```python
from build123d import *

# Parameters (mm, degrees)
BOSS_EXTRUDE1_DEPTH     = 50
SKETCH2_W               = 70
SKETCH2_H               = 26.5
CUT_EXTRUDE1_DEPTH      = 1
CUT_EXTRUDE1_DEPTH_BACK = 26
FILLET1_R               = 2.5
FILLET2_R               = 5
SKETCH3_R               = 1.6
CUT_EXTRUDE2_DEPTH      = 23.0000001
CUT_EXTRUDE2_DEPTH_BACK = 4


with BuildPart() as part:
    # Sketch1 → Boss-Extrude1 (new body, symmetric)
    with BuildSketch(Plane(origin=(0, 0, 0), x_dir=(0, 0, -1), z_dir=(1, 0, 0))):
        with BuildLine():
            Line((-11, 11.5), (11, 11.5))
            ThreePointArc((11, 11.5), (19.131727984, 8.131727984), (22.5, 0))
            Line((22.5, 0), (22.5, -11.5))
            Line((22.5, -11.5), (34.5, -11.5))
            Line((34.5, -11.5), (34.5, -8.5))
            Line((34.5, -8.5), (25, -8.5))
            Line((25, -8.5), (25, 0))
            Line((25, 0), (25, 3.5))
            ThreePointArc((25, 3.5), (22.071067812, 10.571067812), (15, 13.5))
            Line((15, 13.5), (-15, 13.5))
            ThreePointArc((-15, 13.5), (-22.071067812, 10.571067812), (-25, 3.5))
            Line((-25, 3.5), (-25, 0))
            Line((-25, 0), (-25, -8.5))
            Line((-25, -8.5), (-34.5, -8.5))
            Line((-34.5, -8.5), (-34.5, -11.5))
            Line((-34.5, -11.5), (-22.5, -11.5))
            Line((-22.5, -11.5), (-22.5, 0))
            ThreePointArc((-22.5, 0), (-19.131727984, 8.131727984), (-11, 11.5))
        make_face()
    extrude(amount=BOSS_EXTRUDE1_DEPTH, both=True)

    # Sketch2 → Cut-Extrude1 (cut, two sides)
    with BuildSketch(Plane(origin=(0, 13.5, 0), x_dir=(1, 0, 0), z_dir=(0, 1, 0))) as cut_extrude1_sk:
        with Locations((0, 21.25)):
            Rectangle(SKETCH2_W, SKETCH2_H)
        with Locations((0, -21.25)):
            Rectangle(SKETCH2_W, SKETCH2_H)
    extrude(amount=CUT_EXTRUDE1_DEPTH, mode=Mode.SUBTRACT)
    extrude(cut_extrude1_sk.sketch, amount=-CUT_EXTRUDE1_DEPTH_BACK, mode=Mode.SUBTRACT)

    # Fillet1
    fillet1_edges = [part.edges().sort_by_distance(p)[0] for p in [
        (42.5, -8.5, 25),
        (42.5, -8.5, -25),
        (-42.5, -8.5, 25),
        (-42.5, -8.5, -25),
    ]]
    fillet(fillet1_edges, radius=FILLET1_R)

    # Fillet2
    fillet2_edges = [part.edges().sort_by_distance(p)[0] for p in [
        (35, 12.5, -8),
        (35, 12.5, 8),
        (-35, 12.5, 8),
        (-35, 12.5, -8),
    ]]
    fillet(fillet2_edges, radius=FILLET2_R)

    # Sketch3 → Cut-Extrude2 (cut, two sides)
    with BuildSketch(Plane(origin=(0, -8.5, 0), x_dir=(1, 0, 0), z_dir=(0, 1, 0))) as cut_extrude2_sk:
        with Locations((42.5, -31)):
            Circle(SKETCH3_R)
        with Locations((42.5, 31)):
            Circle(SKETCH3_R)
        with Locations((-42.5, 31)):
            Circle(SKETCH3_R)
        with Locations((-42.5, -31)):
            Circle(SKETCH3_R)
    extrude(amount=CUT_EXTRUDE2_DEPTH, mode=Mode.SUBTRACT)
    extrude(cut_extrude2_sk.sketch, amount=-CUT_EXTRUDE2_DEPTH_BACK, mode=Mode.SUBTRACT)


solid = part.part
```
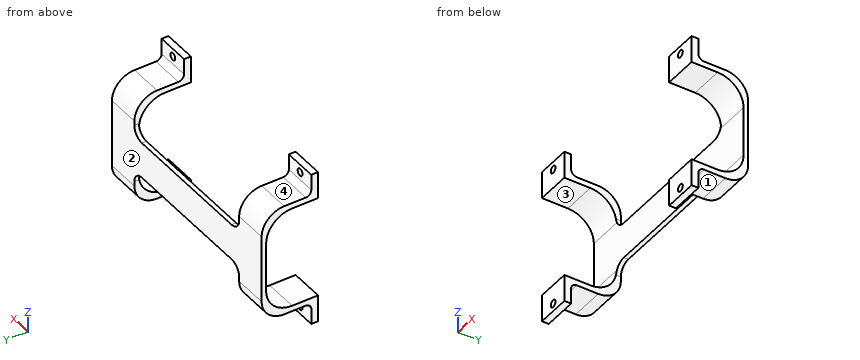
Can you work these out from the model? Positions are in its coordinate system, mm. Face numbers are marked on the shaded views. A direction names the side the tool comes from. Give positions to 0.01 mm unless a question says otherwise; leave off trailing zeros. Loops run counter-clockwise (first coordinate to the right, second up) from the corner with the lowest first, then second, coordinate; pieces in that order, holes last. Notation, with made-up numbers: M 38.25,-23 L 88.25,-23 A12 cw 88.25,-5 Z; hole C 48.5,89 d3. An arc over 180 degrees is marked long. Answer in a Markdown table with one row per item.
1. Suppose I cut it at D-D on x = 38. Write out the boundary of the cut face in (y, z).
Taken from the geometry:
| item | result |
|---|---|
| outline | M -11.5,-34.5 L -8.5,-34.5 L -8.5,-27.5 A2.5 cw -6,-25 L 3.5,-25 A10 ccw 13.5,-15 L 13.5,15 A10 ccw 3.5,25 L -6,25 A2.5 cw -8.5,27.5 L -8.5,34.5 L -11.5,34.5 L -11.5,22.5 L 0,22.5 A11.5 cw 11.5,11 L 11.5,-11 A11.5 cw 0,-22.5 L -11.5,-22.5 Z |
2. Suppose I cut it at C-C on y = -2.25. Write out the boundary of the cut face in (x, z), plus the area to 3 significant figures.
Taken from the geometry:
| item | result |
|---|---|
| outline | M -50,-25 L -35,-25 L -35,-22.5 L -50,-22.5 Z; M -50,22.5 L -35,22.5 L -35,25 L -50,25 Z; M 35,-25 L 50,-25 L 50,-22.5 L 35,-22.5 Z; M 35,22.5 L 50,22.5 L 50,25 L 35,25 Z |
| area | 150 mm² |
3. If I drill on line 1 along Z through (x, y) = (-42.5, -10); line 2 along X through (y, z) = (-10.3, 31); line 3 along X through (y, z) = (-2, 24), over which ranges is the centre line in solid material (lowest first)?
Taken from the geometry:
| item | result |
|---|---|
| line 1 | z = -34.5 to -32.6, -29.4 to -22.5, 22.5 to 29.4, 32.6 to 34.5 |
| line 2 | x = -50 to -44.1, -40.9 to -35, 35 to 40.9, 44.1 to 50 |
| line 3 | x = -50 to -35, 35 to 50 |
4. Suppose I cut it at B-B on z = -31. Write out the boundary of the cut face in (x, y), plus the area to 3 significant figures.
Taken from the geometry:
| item | result |
|---|---|
| outline | M -50,-11.5 L -44.1,-11.5 L -44.1,-8.5 L -50,-8.5 Z; M -40.9,-11.5 L -35,-11.5 L -35,-8.5 L -40.9,-8.5 Z; M 35,-11.5 L 40.9,-11.5 L 40.9,-8.5 L 35,-8.5 Z; M 44.1,-11.5 L 50,-11.5 L 50,-8.5 L 44.1,-8.5 Z |
| area | 70.8 mm² |
5. For pin 1 Ø3.5 at (x, z) = (-42, -32.5) entering from +Y; pin 2 Ø10 at (x, y) = (-39.5, -1.5) entering from +Z; pin 3 Ø5 at (x, y) = (-42.5, 0) entering from -Z; pin 4 Ø12 at (x, z) = (1, 15.5) entering from -Y, each with a flat end and sliding along its axis, tell me the tip position at first contact or that it passes through.
Taken from the geometry:
| item | result |
|---|---|
| pin 1 | stops at y = -8.5 |
| pin 2 | stops at z = 25.05 |
| pin 3 | stops at z = -25 |
| pin 4 | passes through |
6. Which directions (+Z, -Z, +X, -X, +Y, -Y) give clear straight access to the entire face, cutting with the end or side of a thin tool? Please do the marked faces 1, 2, 3 and 4.
Taken from the geometry:
| item | result |
|---|---|
| face 1 | -Z, +X, -X, +Y |
| face 2 | +Z, -Z, +X, -X, +Y |
| face 3 | +X, -X, -Y |
| face 4 | +Z, +X, -X, +Y |
7. Suppose I cut it at A-A on x = -42.5. Write out the boundary of the cut face in (y, z), plus the area to 3 significant figures.
Taken from the geometry:
| item | result |
|---|---|
| outline | M -11.5,-34.5 L -8.5,-34.5 L -8.5,-32.6 L -11.5,-32.6 Z; M -11.5,-29.4 L -8.5,-29.4 L -8.5,-27.5 A2.5 cw -6,-25 L 3.5,-25 A10 ccw 13.5,-15 L 13.5,15 A10 ccw 3.5,25 L -6,25 A2.5 cw -8.5,27.5 L -8.5,29.4 L -11.5,29.4 L -11.5,22.5 L 0,22.5 A11.5 cw 11.5,11 L 11.5,-11 A11.5 cw 0,-22.5 L -11.5,-22.5 Z; M -11.5,32.6 L -8.5,32.6 L -8.5,34.5 L -11.5,34.5 Z |
| area | 269 mm² |
